Source: CAD feature listing. Evaluate the final solid. Frame: model axes, mm. A direction names the side the tool comes from. Give positions to 0.01 mm unless a question says otherwise; leave off trailing zeros. Write each loop counter-clockwise with the first axis right and the second up, starting at its lowest first coordinate (ties: lowest second). Pieces come first, ordered by that corner, then holes. Notation, with made-up numbers: (61, 76.25) -> (81, 76.25) arc R29 cw to (81, 104.25) -> close; hole circle Ø11 at (55.25, 32). An arc over 180 degrees is marked (long way). Use one line per item in the form item = value. Start each with the question number.
(1) Set-up query: faces 4 (the face through (52.5, -5, -16)), 5 (the face through (27.5, 1, -47)), 6 (the face through (32, 0, -28)), 7 (the face through (12.5, -5, -40)), 8 (the face through (32, -6, -18)). Return all of +Z, -Z, +X, -X, +Y, -Y with unobstructed straight access to the full face (end or side cutting, diameter ignored); none if empty.
(2) Material intervals for line 1 along X through (y, z) = (1, -23); line 2 along Z through (x, y) = (32, -2); line 3 along Y through (x, z) = (27.5, -15.1), sorted ascending. Write a range as from..to.
(3) Cut plane B-B, the plane z = -19. Output: boundary loops of the cut face in (x, y), and give its area (3 significant figures).
(4) Cut plane C-C, the plane x = 3.5. Output: boundary loops of the cut face in (y, z), and give its area (3 significant figures).
(5) Cut plane D-D, the plane x = 16.5. Output: boundary loops of the cut face in (y, z).
(6) Cut plane A-A, the plane y = -5.5. Output: boundary loops of the cut face in (x, z).
(7) First-contact query: P1, Ø8.5, axis at x = 37.5, y = -10, coming from the -Z side; P2, Ø1.5, axis at x = 48, y = -2, coming from the +Z side; P3, Ø4.5, axis at y = -3, z = -40.5, coming from the +X side. Flat tips, straight axial feed; report the tip coordinate or a pass-through.
(8) Draft query along X for faces 1 (the face through (27.5, 1, -28)), 2 (the face through (17.878, -14.771, -39.972)), 3 (the face through (32, 1, 0)). Return one class per face: pulls with the +X half, pulls with the -X half, needs draft (parallel to the pull), parting line crosses it, or undercut.
from build123d import *

# Parameters (mm, degrees)
SKETCH1_W           = 65
SKETCH1_H           = 56
SKETCH1_R           = 1.5
SKETCH1_W_2         = 20.5
SKETCH1_H_2         = 20
SKETCH1_H_3         = 10.5
BOSS_EXTRUDE1_DEPTH = 3
SKETCH5_W           = 40
SKETCH5_H           = 4
BOSS_EXTRUDE4_DEPTH = 20
CUT_EXTRUDE1_REACH  = 81.931
SKETCH6_R           = 2.65


with BuildPart() as part:
    # Sketch1 → Boss-Extrude1 (new body)
    with BuildSketch(Plane(origin=(0, 0, 0), x_dir=(1, 0, 0), z_dir=(0, 1, 0))):
        with Locations((32.5, 28)):
            Rectangle(SKETCH1_W, SKETCH1_H)
        with Locations(Location((3.5, 52.5, 0), (0, 0, 270))):
            Circle(SKETCH1_R, mode=Mode.SUBTRACT)
        with Locations(Location((61.5, 52.5, 0), (0, 0, 270))):
            Circle(SKETCH1_R, mode=Mode.SUBTRACT)
        with Locations(Location((61.5, 3.5, 0), (0, 0, 270))):
            Circle(SKETCH1_R, mode=Mode.SUBTRACT)
        with Locations(Location((3.5, 3.5, 0), (0, 0, 270))):
            Circle(SKETCH1_R, mode=Mode.SUBTRACT)
        with Locations((17.25, 28)):
            Rectangle(SKETCH1_W_2, SKETCH1_H_2, mode=Mode.SUBTRACT)
        with Locations((47.75, 28)):
            Rectangle(SKETCH1_W_2, SKETCH1_H_2, mode=Mode.SUBTRACT)
        with Locations((17.25, 47.25)):
            Rectangle(SKETCH1_W_2, SKETCH1_H_3, mode=Mode.SUBTRACT)
        with Locations((47.75, 47.25)):
            Rectangle(SKETCH1_W_2, SKETCH1_H_3, mode=Mode.SUBTRACT)
        with Locations((47.75, 8.75)):
            Rectangle(SKETCH1_W_2, SKETCH1_H_3, mode=Mode.SUBTRACT)
        with Locations((17.25, 8.75)):
            Rectangle(SKETCH1_W_2, SKETCH1_H_3, mode=Mode.SUBTRACT)
    extrude(amount=BOSS_EXTRUDE1_DEPTH)

    # Sketch5 → Boss-Extrude4 (add)
    with BuildSketch(Plane.XZ):
        with Locations((32.5, -16)):
            Rectangle(SKETCH5_W, SKETCH5_H)
        with Locations((32.5, -40)):
            Rectangle(SKETCH5_W, SKETCH5_H)
    extrude(amount=BOSS_EXTRUDE4_DEPTH)

    # Cut-Extrude1: up to this face of the body (flat: up to its plane)
    cut_extrude1_end = Plane(part.part.faces().sort_by_distance((32.5, -8.467497291, -42))[0])
    # Sketch6 → Cut-Extrude1 (cut, up to the picked face)
    with BuildSketch(Plane.XY.offset(-14), mode=Mode.PRIVATE) as cut_extrude1_sk1:
        with Locations((27.5, -10)):
            Circle(SKETCH6_R)
    cut_extrude1_tool1 = split(extrude(cut_extrude1_sk1.sketch, amount=-CUT_EXTRUDE1_REACH, mode=Mode.PRIVATE), bisect_by=cut_extrude1_end, keep=Keep.BOTH, mode=Mode.PRIVATE)
    # Sketch6 → Cut-Extrude1 (cut, up to the picked face)
    with BuildSketch(Plane.XY.offset(-14), mode=Mode.PRIVATE) as cut_extrude1_sk2:
        with Locations((37.5, -10)):
            Circle(SKETCH6_R)
    cut_extrude1_tool2 = split(extrude(cut_extrude1_sk2.sketch, amount=-CUT_EXTRUDE1_REACH, mode=Mode.PRIVATE), bisect_by=cut_extrude1_end, keep=Keep.BOTH, mode=Mode.PRIVATE)
    # Sketch6 → Cut-Extrude1 (cut, up to the picked face)
    with BuildSketch(Plane.XY.offset(-14), mode=Mode.PRIVATE) as cut_extrude1_sk3:
        Polygon((12.5, -9.393398282), (12.5, -20), (23.106601718, -20), align=None)
    cut_extrude1_tool3 = split(extrude(cut_extrude1_sk3.sketch, amount=-CUT_EXTRUDE1_REACH, mode=Mode.PRIVATE), bisect_by=cut_extrude1_end, keep=Keep.BOTH, mode=Mode.PRIVATE)
    # Sketch6 → Cut-Extrude1 (cut, up to the picked face)
    with BuildSketch(Plane.XY.offset(-14), mode=Mode.PRIVATE) as cut_extrude1_sk4:
        Polygon((41.893398282, -20), (52.5, -20), (52.5, -9.393398282), align=None)
    cut_extrude1_tool4 = split(extrude(cut_extrude1_sk4.sketch, amount=-CUT_EXTRUDE1_REACH, mode=Mode.PRIVATE), bisect_by=cut_extrude1_end, keep=Keep.BOTH, mode=Mode.PRIVATE)
    add(cut_extrude1_tool1.solids().sort_by(Axis((27.5, -10, -14), (0, 0, -1)))[0], mode=Mode.SUBTRACT)
    add(cut_extrude1_tool2.solids().sort_by(Axis((37.5, -10, -14), (0, 0, -1)))[0], mode=Mode.SUBTRACT)
    add(cut_extrude1_tool3.solids().sort_by(Axis((16.035534, -16.464466, -14), (0, 0, -1)))[0], mode=Mode.SUBTRACT)
    add(cut_extrude1_tool4.solids().sort_by(Axis((48.964466, -16.464466, -14), (0, 0, -1)))[0], mode=Mode.SUBTRACT)


solid = part.part
Geometry says:
q1.face_4 = +Z, -Z, +X, -Y
q1.face_5 = +Y, -Y
q1.face_6 = +X, -X, -Y
q1.face_7 = +Z, -Z, -X, -Y
q1.face_8 = -Y
q2.line_1 = 0..7, 27.5..37.5, 58..65
q2.line_2 = -42..-38, -18..-14
q2.line_3 = -20..-12.65, -7.35..3
q3.outline = (0, 0) -> (7, 0) -> (7, 3) -> (0, 3) -> close; (27.5, 0) -> (37.5, 0) -> (37.5, 3) -> (27.5, 3) -> close; (58, 0) -> (65, 0) -> (65, 3) -> (58, 3) -> close
q3.area = 72.0 mm^2
q4.outline = (0, -56) -> (3, -56) -> (3, -54) -> (0, -54) -> close; (0, -51) -> (3, -51) -> (3, -5) -> (0, -5) -> close; (0, -2) -> (3, -2) -> (3, 0) -> (0, 0) -> close
q4.area = 150 mm^2
q5.outline = (-13.39, -42) -> (3, -42) -> (3, -38) -> (-13.39, -38) -> close; (-13.39, -18) -> (3, -18) -> (3, -14) -> (-13.39, -14) -> close; (0, -56) -> (3, -56) -> (3, -52.5) -> (0, -52.5) -> close; (0, -3.5) -> (3, -3.5) -> (3, 0) -> (0, 0) -> close
q6.outline = (12.5, -42) -> (52.5, -42) -> (52.5, -38) -> (12.5, -38) -> close; (12.5, -18) -> (52.5, -18) -> (52.5, -14) -> (12.5, -14) -> close
q7.P1 = -42
q7.P2 = -14
q7.P3 = 52.5
q8.face_1 = undercut
q8.face_2 = pulls with the -X half
q8.face_3 = needs draft
